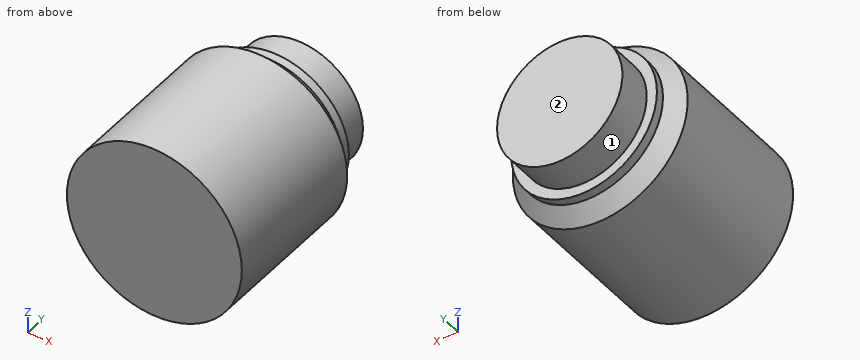
from build123d import *

# Parameters (mm, degrees)
F0_W    = 0.7
F0_H    = 0.6
F2_SIZE = 0.99999


# Not quite as in the source:
# - a fillet or chamfer is up to 0.001 mm smaller than in the source, because OpenCascade refuses the exact size


with BuildPart() as f1:
    # F0 (on Top) → F1 (revolve)
    with BuildSketch(Plane.XY):
        with Locations((4.65, 11.7)):
            Rectangle(F0_W, F0_H)
        Polygon((0, 14.4), (0, 0), (6, 0), (6, 11.4), (5, 11.4), (4.3, 11.4), (4.3, 12), (4.3, 14.4), align=None)
    revolve(axis=Axis((0, 7.2, 0), (0, 1, 0)))

    # F2 (size 1 in the source; OpenCascade refuses exactly that, so slightly less here)
    f2_edges = [f1.edges().sort_by_distance(p)[0] for p in [
        (-6, 11.4, 0),
    ]]
    chamfer(f2_edges, length=F2_SIZE)


solid = f1.part
Check sheet for the modelled part. Datum: model origin and axes. Units: mm. Face numbers are marked on the shaded views. Give positions to 0.01 mm unless a question says otherwise; leave off trailing zeros. Write each loop counter-clockwise with the first axis right and the second up, starting at its lowest first coordinate (ties: lowest second). Pieces come first, ordered by that corner, then holes. Notation, with made-up numbers: (7.25, -35.75) -> (46.25, -35.75) arc R29 cw to (46.25, -3.75) -> close; hole circle Ø1 at (28, 73). An arc over 180 degrees is marked (long way). Use one line per item in the form item = value. Start each with the question number.
1. Thickness scan on line 1 along Z through (x, y) = (-1, 5.5); line 2 along Y through (x, z) = (5.25, 1); line 3 along X through (y, z) = (7.75, 2.25). Record the ranges inside material, lowest first. Write a range as from..to.
2. Mould release check, pull along X, two halves, no side actions. Record for the marked faces 1 and 2: pulls with the +X half, pulls with the -X half, needs draft (parallel to the pull), parting line crosses it, or undercut.
3. Section check D-D (y = 10.75). Record the cut outline in (x, z), and give its area (3 significant figures).
4. Section check C-C (y = 8.5). Record the cut outline in (x, z), and give its area (3 significant figures).
5. Go/stop test with a flat-tipped pin: P1, Ø1, axis at x = -2, z = -4.5, coming from the +Y side. Record where the tip stops, or that it passes through.
Conclusion:
q1.line_1 = -5.92..5.92
q1.line_2 = 0..11.06
q1.line_3 = -5.56..5.56
q2.face_1 = parting line crosses it
q2.face_2 = needs draft
q3.outline = circle Ø11.3 at (0, 0)
q3.area = 100 mm²
q4.outline = circle Ø12 at (0, 0)
q4.area = 113 mm²
q5.P1 = 12
